Work out the finished part from the listing and answer in its coordinate system (mm). Face numbers are marked on the shaded views. A direction names the side the tool comes from. Coordinates: 2 decimals unless noted, no trailing zeros. Order: outer loops, then holes, each group sorted by start corner. A loop starts at its lowest first (then second) coordinate and runs counter-clockwise, first axis right, second up. Notation, with made-up numbers: M 71,44.25 L 109,44.25 A37 cw 109,83.25 Z; hole C 8,44.5 d7. An arc over 180 degrees is marked long. Use a Markdown table: item, result.
from build123d import *

# Parameters (mm, degrees)
F0_R     = 20
F1_DEPTH = 38.5
F2_W     = 40
F2_H     = 43
F3_DEPTH = 43
F4_R     = 20
F4_R_2   = 11
F5_DEPTH = 25
F6_R     = 5


with BuildPart() as f1:
    # F0 (on Front) → F1 (new body)
    with BuildSketch(Plane.XZ):
        Circle(F0_R)
    extrude(amount=F1_DEPTH)

    # F2 (on face) → F3 (join)
    with BuildSketch(Plane(origin=(0, 0, 0), x_dir=(-1, 0, 0), z_dir=(0, 1, 0))):
        Rectangle(F2_W, F2_H)
    extrude(amount=F3_DEPTH)

    # F4 (on face) → F5 (cut)
    with BuildSketch(Plane.XZ):
        Circle(F4_R)
        Circle(F4_R_2, mode=Mode.SUBTRACT)
    extrude(amount=F5_DEPTH, mode=Mode.SUBTRACT)

    # F6
    f6_edges = [f1.edges().sort_by_distance(p)[0] for p in [
        (-20, -38.5, 0),
    ]]
    fillet(f6_edges, radius=F6_R)


solid = f1.part
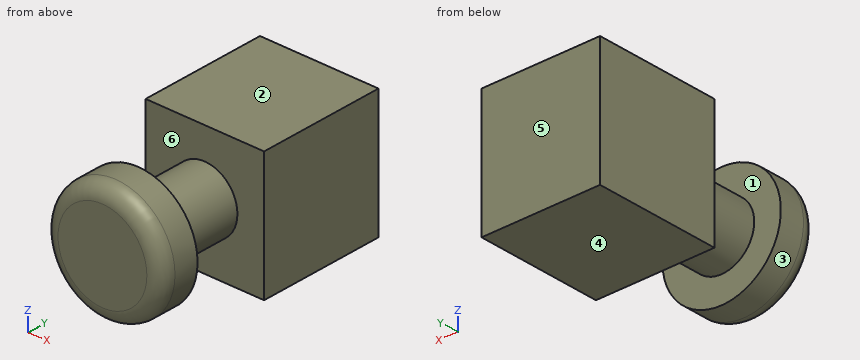
1. Flat-ended cylindrical pins translate along their axes: P1, Ø6, axis at x = 3, z = 16.5, coming from the -Y side; P2, Ø1, axis at x = -10, y = -20, coming from the +Z side. Find the tip coordinate at first contact, or state that the pin passes through.
Answers below:
| item | result |
|---|---|
| P1 | y = -38.5 |
| P2 | z = 5.55 |
2. Find the intervals of material crossed by probe 1 along Y at (x, z) = (13, -7); probe 2 along Y at (x, z) = (16.5, -14.5); probe 3 along Y at (x, z) = (16, -1), in increasing order.
Answers below:
| item | result |
|---|---|
| probe 1 | -38.5 to -25, 0 to 43 |
| probe 2 | 0 to 43 |
| probe 3 | -38.39 to -25, 0 to 43 |
3. For a pull along Y with two mould halves and no side action, classify the marked faces 4, 5 and 6 as +Y half, -Y half, draft (parallel to the pull), parting line (faces both ways), or undercut.
Answers below:
| item | result |
|---|---|
| face 4 | draft |
| face 5 | +Y half |
| face 6 | undercut |
4. For the marked faces 1, 2 and 3, determine the directions among +Z, -Z, +X, -X, +Y, -Y from which every point of the face is accessible in a straight line to the end or side of a thin tool.
Answers below:
| item | result |
|---|---|
| face 1 | none |
| face 2 | +Z, +X, -X, +Y, -Y |
| face 3 | -Y |
5. Section B-B on x = 0 is taken. Determine the outline of the cut face in (y, z), then the cut area to 3 significant figures.
Answers below:
| item | result |
|---|---|
| outline | M -38.5,-15 A5 ccw -33.5,-20 L -25,-20 L -25,-11 L 0,-11 L 0,-21.5 L 43,-21.5 L 43,21.5 L 0,21.5 L 0,11 L -25,11 L -25,20 L -33.5,20 A5 ccw -38.5,15 Z |
| area | 2,930 mm² |
6. Section C-C on y = -4.5 is taken. Determine the outline of the cut face in (x, z).
Answers below:
| item | result |
|---|---|
| outline | C 0,0 d22 |
7. Section A-A on z = 0 is taken. Determine the outline of the cut face in (x, y), then the cut area to 3 significant figures.
Answers below:
| item | result |
|---|---|
| outline | M -20,-33.5 A5 ccw -15,-38.5 L 15,-38.5 A5 ccw 20,-33.5 L 20,-25 L 11,-25 L 11,0 L 20,0 L 20,43 L -20,43 L -20,0 L -11,0 L -11,-25 L -20,-25 Z |
| area | 2,800 mm² |
